```python
from build123d import *

# Parameters (mm, degrees)
EXTRUDE_1_DEPTH     = 10
EXTRUDE_2_DEPTH     = 10
FILLET_1_R          = 5
SKETCH_3_R          = 5
CUT_EXTRUDE_1_DEPTH = 10
SKETCH_4_R          = 2
CUT_EXTRUDE_2_DEPTH = 10


with BuildPart() as part:
    # 草图1 → 凸台-拉伸1 (new body)
    with BuildSketch(Plane(origin=(0, 0, 0), x_dir=(0, 0, -1), z_dir=(1, 0, 0))):
        with BuildLine():
            ThreePointArc((-7.942884534, 22.647529341), (-9.184402377, 22.17310878), (-10.397754058, 21.630689091))
            ThreePointArc((-10.397754058, 21.630689091), (-12.397305949, 24.184674774), (-15.156649968, 25.889688329))
            ThreePointArc((-15.156649968, 25.889688329), (-15.674956941, 25.579204931), (-16.186906117, 25.258346549))
            ThreePointArc((-16.186906117, 25.258346549), (-15.920443886, 22.02569307), (-14.552603542, 19.084594053))
            ThreePointArc((-14.552603542, 19.084594053), (-15.58675316, 18.249743174), (-16.573102281, 17.358925105))
            ThreePointArc((-16.573102281, 17.358925105), (-19.264014116, 19.170014316), (-22.41518439, 19.938894372))
            ThreePointArc((-22.41518439, 19.938894372), (-22.812178968, 19.48344145), (-23.199920874, 19.020085999))
            ThreePointArc((-23.199920874, 19.020085999), (-21.947555371, 16.027991201), (-19.737812321, 13.653525728))
            ThreePointArc((-19.737812321, 13.653525728), (-20.463363944, 12.539965553), (-21.126159781, 11.387948582))
            ThreePointArc((-21.126159781, 11.387948582), (-24.245026361, 12.278859291), (-27.479564388, 12.036342512))
            ThreePointArc((-27.479564388, 12.036342512), (-27.716385975, 11.480502971), (-27.941965733, 10.920006912))
            ThreePointArc((-27.941965733, 10.920006912), (-25.82628722, 8.46135788), (-22.990946508, 6.885955175))
            ThreePointArc((-22.990946508, 6.885955175), (-23.33687809, 5.602688733), (-23.611241567, 4.302240308))
            ThreePointArc((-23.611241567, 4.302240308), (-26.852766501, 4.185763967), (-29.854053162, 2.955589584))
            ThreePointArc((-29.854053162, 2.955589584), (-29.907520012, 2.353772872), (-29.948856303, 1.751001464))
            ThreePointArc((-29.948856303, 1.751001464), (-27.176962132, 0.066467896), (-23.993566664, -0.555660648))
            ThreePointArc((-23.993566664, -0.555660648), (-23.92601601, -1.883018297), (-23.785090519, -3.204601222))
            ThreePointArc((-23.785090519, -3.204601222), (-26.831970761, -4.317063099), (-29.306219208, -6.414477044))
            ThreePointArc((-29.306219208, -6.414477044), (-29.171097612, -7.003360916), (-29.024144152, -7.589404208))
            ThreePointArc((-29.024144152, -7.589404208), (-25.867366639, -8.334928429), (-22.647529341, -7.942884534))
            ThreePointArc((-22.647529341, -7.942884534), (-22.17310878, -9.184402377), (-21.630689091, -10.397754058))
            ThreePointArc((-21.630689091, -10.397754058), (-24.184674774, -12.397305949), (-25.889688329, -15.156649968))
            ThreePointArc((-25.889688329, -15.156649968), (-25.579204931, -15.674956941), (-25.258346549, -16.186906117))
            ThreePointArc((-25.258346549, -16.186906117), (-22.02569307, -15.920443886), (-19.084594053, -14.552603542))
            ThreePointArc((-19.084594053, -14.552603542), (-18.249743174, -15.58675316), (-17.358925105, -16.573102281))
            ThreePointArc((-17.358925105, -16.573102281), (-19.170014316, -19.264014116), (-19.938894372, -22.41518439))
            ThreePointArc((-19.938894372, -22.41518439), (-19.48344145, -22.812178968), (-19.020085999, -23.199920874))
            ThreePointArc((-19.020085999, -23.199920874), (-16.027991201, -21.947555371), (-13.653525728, -19.737812321))
            ThreePointArc((-13.653525728, -19.737812321), (-12.539965553, -20.463363944), (-11.387948582, -21.126159781))
            ThreePointArc((-11.387948582, -21.126159781), (-12.278859291, -24.245026361), (-12.036342512, -27.479564388))
            ThreePointArc((-12.036342512, -27.479564388), (-11.480502971, -27.716385975), (-10.920006912, -27.941965733))
            ThreePointArc((-10.920006912, -27.941965733), (-8.46135788, -25.82628722), (-6.885955175, -22.990946508))
            ThreePointArc((-6.885955175, -22.990946508), (-5.602688733, -23.33687809), (-4.302240308, -23.611241567))
            ThreePointArc((-4.302240308, -23.611241567), (-4.185763967, -26.852766501), (-2.955589584, -29.854053162))
            ThreePointArc((-2.955589584, -29.854053162), (-2.353772872, -29.907520012), (-1.751001464, -29.948856303))
            ThreePointArc((-1.751001464, -29.948856303), (-0.066467896, -27.176962132), (0.555660648, -23.993566664))
            ThreePointArc((0.555660648, -23.993566664), (1.883018297, -23.92601601), (3.204601222, -23.785090519))
            ThreePointArc((3.204601222, -23.785090519), (4.317063099, -26.831970761), (6.414477044, -29.306219208))
            ThreePointArc((6.414477044, -29.306219208), (7.003360916, -29.171097612), (7.589404208, -29.024144152))
            ThreePointArc((7.589404208, -29.024144152), (8.334928429, -25.867366639), (7.942884534, -22.647529341))
            ThreePointArc((7.942884534, -22.647529341), (9.184402377, -22.17310878), (10.397754058, -21.630689091))
            ThreePointArc((10.397754058, -21.630689091), (12.397305949, -24.184674774), (15.156649968, -25.889688329))
            ThreePointArc((15.156649968, -25.889688329), (15.674956941, -25.579204931), (16.186906117, -25.258346549))
            ThreePointArc((16.186906117, -25.258346549), (15.920443886, -22.02569307), (14.552603542, -19.084594053))
            ThreePointArc((14.552603542, -19.084594053), (15.58675316, -18.249743174), (16.573102281, -17.358925105))
            ThreePointArc((16.573102281, -17.358925105), (19.264014116, -19.170014316), (22.41518439, -19.938894372))
            ThreePointArc((22.41518439, -19.938894372), (22.812178968, -19.48344145), (23.199920874, -19.020085999))
            ThreePointArc((23.199920874, -19.020085999), (21.947555371, -16.027991201), (19.737812321, -13.653525728))
            ThreePointArc((19.737812321, -13.653525728), (20.463363944, -12.539965553), (21.126159781, -11.387948582))
            ThreePointArc((21.126159781, -11.387948582), (24.245026361, -12.278859291), (27.479564388, -12.036342512))
            ThreePointArc((27.479564388, -12.036342512), (27.716385975, -11.480502971), (27.941965733, -10.920006912))
            ThreePointArc((27.941965733, -10.920006912), (25.82628722, -8.46135788), (22.990946508, -6.885955175))
            ThreePointArc((22.990946508, -6.885955175), (23.33687809, -5.602688733), (23.611241567, -4.302240308))
            ThreePointArc((23.611241567, -4.302240308), (26.852766501, -4.185763967), (29.854053162, -2.955589584))
            ThreePointArc((29.854053162, -2.955589584), (29.907520012, -2.353772872), (29.948856303, -1.751001464))
            ThreePointArc((29.948856303, -1.751001464), (27.176962132, -0.066467896), (23.993566664, 0.555660648))
            ThreePointArc((23.993566664, 0.555660648), (23.92601601, 1.883018297), (23.785090519, 3.204601222))
            ThreePointArc((23.785090519, 3.204601222), (26.831970761, 4.317063099), (29.306219208, 6.414477044))
            ThreePointArc((29.306219208, 6.414477044), (29.171097612, 7.003360916), (29.024144152, 7.589404208))
            ThreePointArc((29.024144152, 7.589404208), (25.867366639, 8.334928429), (22.647529341, 7.942884534))
            ThreePointArc((22.647529341, 7.942884534), (22.17310878, 9.184402377), (21.630689091, 10.397754058))
            ThreePointArc((21.630689091, 10.397754058), (24.184674774, 12.397305949), (25.889688329, 15.156649968))
            ThreePointArc((25.889688329, 15.156649968), (25.579204931, 15.674956941), (25.258346549, 16.186906117))
            ThreePointArc((25.258346549, 16.186906117), (22.02569307, 15.920443886), (19.084594053, 14.552603542))
            ThreePointArc((19.084594053, 14.552603542), (18.249743174, 15.58675316), (17.358925105, 16.573102281))
            ThreePointArc((17.358925105, 16.573102281), (19.170014316, 19.264014116), (19.938894372, 22.41518439))
            ThreePointArc((19.938894372, 22.41518439), (19.48344145, 22.812178968), (19.020085999, 23.199920874))
            ThreePointArc((19.020085999, 23.199920874), (16.027991201, 21.947555371), (13.653525728, 19.737812321))
            ThreePointArc((13.653525728, 19.737812321), (12.539965553, 20.463363944), (11.387948582, 21.126159781))
            ThreePointArc((11.387948582, 21.126159781), (12.278859291, 24.245026361), (12.036342512, 27.479564388))
            ThreePointArc((12.036342512, 27.479564388), (11.480502971, 27.716385975), (10.920006912, 27.941965733))
            ThreePointArc((10.920006912, 27.941965733), (8.46135788, 25.82628722), (6.885955175, 22.990946508))
            ThreePointArc((6.885955175, 22.990946508), (5.602688733, 23.33687809), (4.302240308, 23.611241567))
            ThreePointArc((4.302240308, 23.611241567), (4.185763967, 26.852766501), (2.955589584, 29.854053162))
            ThreePointArc((2.955589584, 29.854053162), (2.353772872, 29.907520012), (1.751001464, 29.948856303))
            ThreePointArc((1.751001464, 29.948856303), (0.066467896, 27.176962132), (-0.555660648, 23.993566664))
            ThreePointArc((-0.555660648, 23.993566664), (-1.883018297, 23.92601601), (-3.204601222, 23.785090519))
            ThreePointArc((-3.204601222, 23.785090519), (-4.317063099, 26.831970761), (-6.414477044, 29.306219208))
            ThreePointArc((-6.414477044, 29.306219208), (-7.003360916, 29.171097612), (-7.589404208, 29.024144152))
            ThreePointArc((-7.589404208, 29.024144152), (-8.334928429, 25.867366639), (-7.942884534, 22.647529341))
        make_face()
    extrude(amount=EXTRUDE_1_DEPTH)

    # 草图2 → 凸台-拉伸2 (add)
    with BuildSketch(Plane(origin=(10, 0, 0), x_dir=(0, 0, -1), z_dir=(1, 0, 0))):
        Polygon((2.076731947, 90.114855515), (-4.984586669, 0.392295479), (4.984586669, -0.392295479), (12.045905284, 89.330264557), align=None)
    extrude(amount=-EXTRUDE_2_DEPTH)

    # 圆角1
    fillet_1_edges = [part.edges().sort_by_distance(p)[0] for p in [
        (5, 89.330264557, -12.045905284),
        (5, 90.114855515, -2.076731947),
    ]]
    fillet(fillet_1_edges, radius=FILLET_1_R - 0.0001)  # a hair under: the kernel refuses the full size

    # 草图3 → 切除-拉伸1 (cut)
    with BuildSketch(Plane(origin=(10, 0, 0), x_dir=(0, 0, -1), z_dir=(1, 0, 0))):
        Circle(SKETCH_3_R)
    extrude(amount=-CUT_EXTRUDE_1_DEPTH, mode=Mode.SUBTRACT)

    # 草图4 → 切除-拉伸2 (cut)
    with BuildSketch(Plane(origin=(10, 0, 0), x_dir=(0, 0, -1), z_dir=(1, 0, 0))):
        with Locations((6.669023137, 84.737973367)):
            Circle(SKETCH_4_R)
    extrude(amount=-CUT_EXTRUDE_2_DEPTH, mode=Mode.SUBTRACT)


solid = part.part
```
CAD build for the part. Positions are in the model's coordinates, mm. A direction names the side the tool comes from. Coordinates: 2 decimals unless noted, no trailing zeros. Order: outer loops, then holes, each group sorted by start corner. A loop starts at its lowest first (then second) coordinate and runs counter-clockwise, first axis right, second up.
(1) Saw through at B-B, the plane y = 52.5. Write the cut outline in (x, z).
Solution:
outline: (0, -9.15) - (10, -9.15) - (10, 0.88) - (0, 0.88) - close
(2) Drill centre lines: L1, parallel to Z at x = 4.25, y = -3; L2, parallel to Z at x = 6.5, y = 25; L3, parallel to Y at x = 8.5, z = -19. Where is each one in solid material? Low to high.
Solution:
L1: z = -29.78 to -4, 4 to 23.81
L2: z = -12.32 to -7.86, -6.98 to 3.05, 3.5 to 8.34, 13.45 to 16.21
L3: y = -19.05 to 14.66, 18.9 to 23.2
(3) Mould opens along Y. For faces 4 (the face through (10, 4, -6)), 5 (the face through (4.93, 25.86, -8.49)), 6 (the face through (4.93, 19.15, 19.22)) say: released by +Y, released by -Y, zero draft, split by the parting line, or undercut.
Solution:
face 4: zero draft
face 5: undercut
face 6: released by +Y
(4) Pin check, flat tips, straight feed: pin 1 Ø4 at (x, y) = (6, 57) entering from +Z; pin 2 Ø5 at (x, z) = (7, 19.5) entering from -Y; pin 3 Ø6 at (x, y) = (4.5, 54) entering from +Z; pin 4 Ø6 at (y, z) = (0, 0) entering from +X. Stop position of each tip, or through.
Solution:
pin 1: stops at z = 0.69
pin 2: stops at y = -23.2
pin 3: stops at z = 1
pin 4: passes through
(5) Which spindle directions (+Z, -Z, +X, -X, +Y, -Y) get a long thin tool onto all of the face, cutting with end or side? Do faces 1 (the face through (4.93, -25.86, 8.49)), 2 (the face through (4.93, -8.332, 25.913)), 3 (the face through (5, 0, -27)). Say none if no direction does.
Solution:
face 1: +X, -X, -Y
face 2: +X, -X
face 3: -Z, +X, -X
(6) Saw through at A-A, the plane x = 4.25. Count the separate pieces of the cut face and the enclosed holes in it, and give its area (3 significant figures).
Solution:
separate pieces: 1
enclosed holes: 2
area: 2,810 mm2
